from build123d import *

# Parameters (mm, degrees)
SKETCH1_R           = 1.22148615
BOSS_EXTRUDE1_DEPTH = 2.54


with BuildPart() as part:
    # Sketch1 → Boss-Extrude1 (new body)
    with BuildSketch(Plane(origin=(0, 0, 0), x_dir=(1, 0, 0), z_dir=(0, 1, 0))):
        with BuildLine():
            Line((-444.533071271, -69.006399848), (-459.545623253, -81.603426679))
            ThreePointArc((-459.545623253, -81.603426679), (-462.948071271, -88.9), (-459.545623253, -96.196573321))
            Line((-459.545623253, -96.196573321), (-444.533071271, -108.793600152))
            Line((-444.533071271, -108.793600152), (-444.533071271, -69.006399848))
        make_face()
        with Locations((-453.423071271, -88.9)):
            Circle(SKETCH1_R, mode=Mode.SUBTRACT)
    extrude(amount=BOSS_EXTRUDE1_DEPTH)


solid = part.part
The model under review builds one solid part; all positions refer to its coordinate system, in mm. Coordinates: 2 decimals unless noted, no trailing zeros. Loops run counter-clockwise (first coordinate to the right, second up) from the corner with the lowest first, then second, coordinate; pieces in that order, holes last.
(1) Consider section A-A, the plane y = 2.05. Give the boundary of the cut face in (x, z) (3 decimals).
Determined:
outline: (-459.546, 81.603) - (-444.533, 69.006) - (-444.533, 108.794) - (-459.546, 96.197) arc R9.525 ccw to start; hole circle Ø2.443 at (-453.423, 88.9)
(2) Consider section D-D, the plane z = 83.5. Give the boundary of the cut face in (x, y), plus the area to 3 significant figures.
Determined:
outline: (-461.27, 0) - (-444.53, 0) - (-444.53, 2.54) - (-461.27, 2.54) - close
area: 42.5 mm2
(3) Draft analysis for pull direction X (two halves, no side actions). For faces 1 (the cylindrical face through (-462.947, 1.252, 88.784)), 2 (the cylindrical face through (-452.26, 1.25, 88.53)), 3 (the flat face through (-452, 2.54, 89)), state which applies: +X half, -X half, draft (parallel to the pull), parting line (faces both ways), or undercut.
Determined:
face 1: -X half
face 2: undercut
face 3: draft
(4) Insertion check: P1, Ø2, axis at x = -453.42, z = 88.9, coming from the +Y side; P2, Ø1, axis at y = 0.5, z = 86.5, coming from the -X side. Each pin has a flat end and moves straight along its axis. Give the tip position at first contact, or say it passes through.
Determined:
P1: passes through
P2: stops at x = -462.76
(5) Wall thickness on L1, parallel to X at y = 2, z = 88.9; L2, parallel to X at y = 2.2, z = 89.5; L3, parallel to X at y = 1.5, z = 104: over which ranges is each line inside the solid? List them lowest first.
Determined:
L1: x = -462.95 to -454.64, -452.2 to -444.53
L2: x = -462.93 to -454.49, -452.36 to -444.53
L3: x = -450.25 to -444.53
(6) Consider section C-C, the plane x = -458. Give the boundary of the cut face in (y, z), plus the area to 3 significant figures.
Determined:
outline: (0, 80.31) - (2.54, 80.31) - (2.54, 97.49) - (0, 97.49) - close
area: 43.7 mm2
(7) Consider section B-B, the plane z = 88.9. Give the boundary of the cut face in (x, y), plus the area to 3 significant figures.
Determined:
outline: (-462.95, 0) - (-454.64, 0) - (-454.64, 2.54) - (-462.95, 2.54) - close; (-452.2, 0) - (-444.53, 0) - (-444.53, 2.54) - (-452.2, 2.54) - close
area: 40.6 mm2
